Geometry check sheet. Reference: drawing and pictorial views, mm from the part's lowest x, y, z. A direction names the side the tool comes from. Round coordinates to 2 decimals unless told otherwise and drop trailing zeros. Loops run counter-clockwise (first coordinate to the right, second up) from the corner with the lowest first, then second, coordinate; pieces in that order, holes last. Notation, with made-up numbers: (74.5, 84.5) - (92.5, 84.5) arc R25 cw to (92.5, 101.5) - close; hole circle Ø7 at (57.25, 14.5). An arc over 180 degrees is marked (long way). Put each result on its own line as item: value. Start each with the question number.
Item 1: Section check A-A, the plane x = 45. Record the cut outline in (y, z) (1 decimal).
Item 2: Tool access check on the marked faces 4, 5 and 6. Record the directions out of +Z, -Z, +X, -X, +Y, -Y that give a thin tool (end or side, any length) a straight path to the whole face; none if there is none.
Item 3: Section check C-C, the plane z = 7.5. Record the cut outline in (x, y) (1 decimal).
Item 4: Gauge pin test, flat ends, axial feed: pin 1 Ø3 at (y, z) = (6.5, 4.5) entering from +X; pin 2 Ø4 at (y, z) = (7, 42.5) entering from -X; pin 3 Ø1 at (x, y) = (45.5, 3) entering from +Z (1 decimal); pin 4 Ø4 at (x, y) = (49, 1) entering from -Z. Record the tip position at first contact, or that the pin passes through.
Item 5: Draft check along Z on the marked faces 1, 2 and 3. Enter one of: pulls with the +Z half, pulls with the -Z half, needs draft (parallel to the pull), parting line crosses it, or undercut.
Item 6: Material ranges on line 1 along Y through (x, z) = (44.5, 57.5); line 2 along Z through (x, y) = (54.5, 4) (1 decimal); line 3 along Z through (x, y) = (65, 3) (1 decimal), recorded low to high.
Item 7: Section check D-D, the plane x = 85. Record the cut outline in (y, z) (1 decimal).
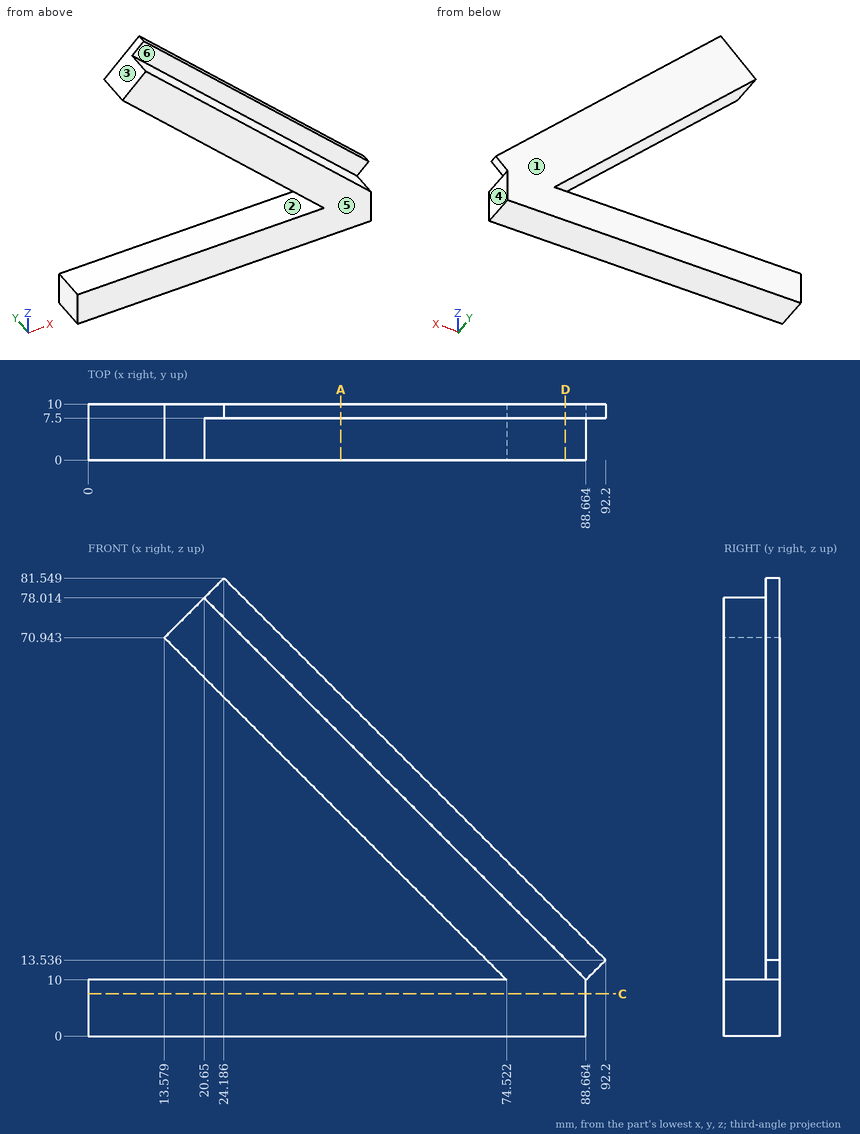
Check result:
1. outline: (0, 0) - (10, 0) - (10, 10) - (0, 10) - close; (0, 39.5) - (10, 39.5) - (10, 60.7) - (7.5, 60.7) - (7.5, 53.7) - (0, 53.7) - close
2. face 4: -Z, +X, +Y, -Y
2. face 5: +Z, -Z, +X, -X, -Y
2. face 6: +Z, +X, -Y
3. outline: (0, 0) - (88.7, 0) - (88.7, 10) - (0, 10) - close
4. pin 1: x = 88.66
4. pin 2: x = 40.02
4. pin 3: z = 53.7
4. pin 4: z = 0
5. face 1: needs draft
5. face 2: undercut
5. face 3: pulls with the +Z half
6. line 1: 7.5 to 10
6. line 2: 0 to 10, 30 to 44.2
6. line 3: 0 to 10, 19.5 to 33.7
7. outline: (0, 0) - (10, 0) - (10, 20.7) - (7.5, 20.7) - (7.5, 13.7) - (0, 13.7) - close
